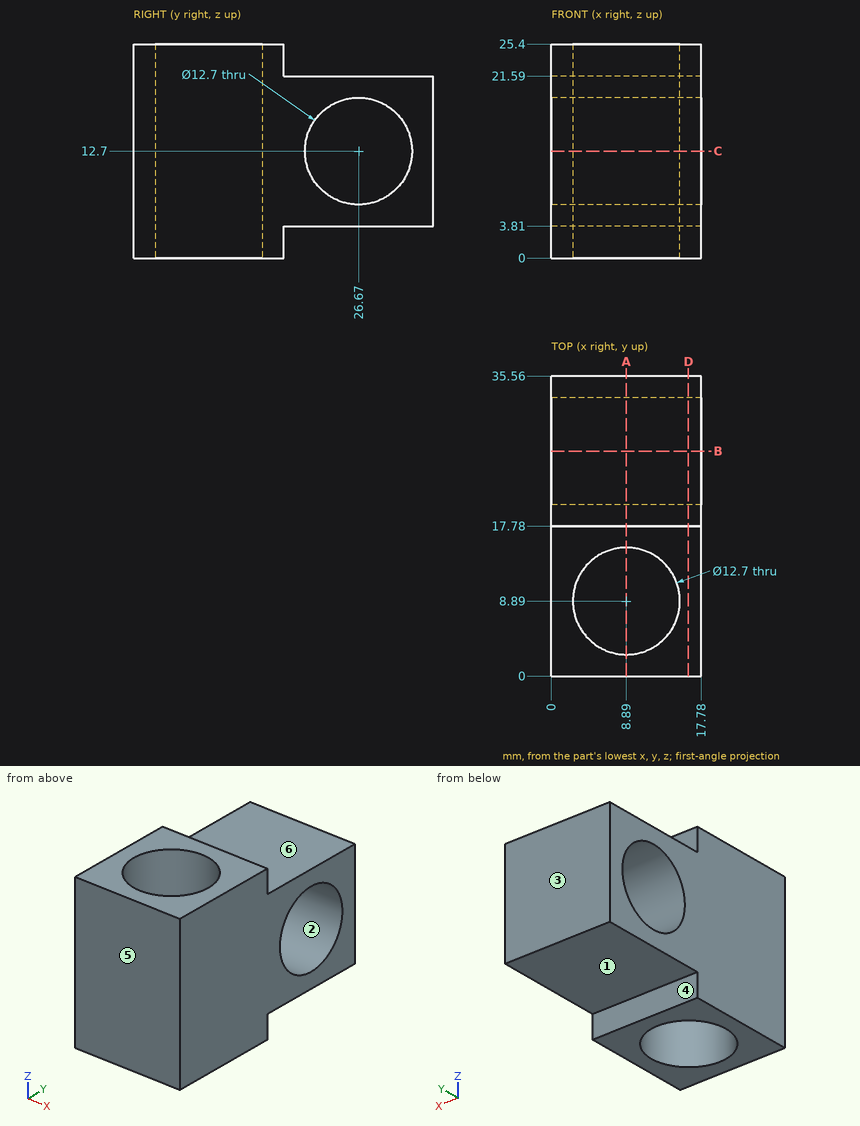
Source: three-view drawing plus pictorial views. Frame: mm from the lowest corner of the part. A direction names the side the tool comes from. Coordinates: 2 decimals unless noted, no trailing zeros. Order: outer loops, then holes, each group sorted by start corner. A loop starts at its lowest first (then second) coordinate and runs counter-clockwise, first axis right, second up. Notation, with made-up numbers: (-18, -32.75) -> (25, -32.75) arc R22 ccw to (25, 3.25) -> close; hole circle Ø11 at (8, 88.25). An arc over 180 degrees is marked (long way). Write item = value, one per line.
(1) Cut plane A-A on x = 8.89. Return loops of the section in (y, z), plus the area to 3 significant figures.
Solved:
outline = (0, 0) -> (2.54, 0) -> (2.54, 25.4) -> (0, 25.4) -> close; (15.24, 0) -> (17.78, 0) -> (17.78, 3.81) -> (35.56, 3.81) -> (35.56, 21.59) -> (17.78, 21.59) -> (17.78, 25.4) -> (15.24, 25.4) -> close; hole circle Ø12.7 at (26.67, 12.7)
area = 318 mm²
(2) Cut plane C-C on z = 12.7. Return loops of the section in (x, y), plus the area to 3 significant figures.
Solved:
outline = (0, 0) -> (17.78, 0) -> (17.78, 20.32) -> (0, 20.32) -> close; (0, 33.02) -> (17.78, 33.02) -> (17.78, 35.56) -> (0, 35.56) -> close; hole circle Ø12.7 at (8.89, 8.89)
area = 280 mm²
(3) Access query for the marked faces 4, 5 and 6. Directions: +Z, -Z, +X, -X, +Y, -Y. A direction counts if a zero-diameter tool reaches every point of the face in a straight line with its end or side. Return the directions, or none.
Solved:
face_4 = -Z, +X, -X, +Y
face_5 = +Z, -Z, +X, -X, -Y
face_6 = +Z, +X, -X, +Y
(4) Cut plane B-B on y = 26.67. Return loops of the section in (x, z).
Solved:
outline = (0, 3.81) -> (17.78, 3.81) -> (17.78, 6.35) -> (0, 6.35) -> close; (0, 19.05) -> (17.78, 19.05) -> (17.78, 21.59) -> (0, 21.59) -> close
(5) Pull-direction query (Z, two-part tool) for the marked faces 1, 2 and 3; classes: pulls with the +Z half, pulls with the -Z half, needs draft (parallel to the pull), parting line crosses it, or undercut.
Solved:
face_1 = pulls with the -Z half
face_2 = undercut
face_3 = needs draft
(6) Pin query (flat end, axial travel): pin 1 Ø3 at (x, z) = (8.5, 24.5) entering from +Y; pin 2 Ø5 at (y, z) = (9, 10.5) entering from -X; pin 3 Ø9 at (x, y) = (7.5, 25) entering from +Z. Return the tip coordinate at first contact, or that it passes through.
Solved:
pin_1 = 17.78
pin_2 = 0
pin_3 = 21.59
(7) Cut plane D-D on x = 16.25. Return loops of the section in (y, z), plus the area to 3 significant figures.
Solved:
outline = (0, 0) -> (17.78, 0) -> (17.78, 3.81) -> (35.56, 3.81) -> (35.56, 21.59) -> (17.78, 21.59) -> (17.78, 25.4) -> (0, 25.4) -> close; hole circle Ø12.7 at (26.67, 12.7)
area = 641 mm²
(8) Line query: line 1 (X direction, y = 9, z = 23.25); line 2 (Y direction, x = 12.25, z = 7.25); line 3 (Z direction, x = 6, y = 26.67). Output: solid intervals per line, ascending.
Solved:
line_1 = 0 to 2.54, 15.24 to 17.78
line_2 = 0 to 3.5, 14.28 to 23.41, 29.93 to 35.56
line_3 = 3.81 to 6.35, 19.05 to 21.59
